from build123d import *

# Parameters (mm, degrees)
BOSS_EXTRUDE1_DEPTH    = 4.75
CUT_EXTRUDE1_REACH     = 11.471
CUT_EXTRUDE2_DEPTH     = 0.85
SKETCH6_W              = 0.8
SKETCH6_H              = 2
CUT_EXTRUDE3_DEPTH     = 0.85
SKETCH7_W              = 1.05
SKETCH7_H              = 0.85
BOSS_EXTRUDE2_DEPTH    = 1
SKETCHED_START         = 1.85
SKETCHED_BEND1_DEPTH   = 1.05
SKETCHED_BEND1_2_DEPTH = 1.05
BOSS_EXTRUDE3_DEPTH    = 0.85


# Read off the part's stored shape, not the designer's step: Sketched Bend1
with BuildPart() as part:
    # Sketch1 → Boss-Extrude1 (new body)
    with BuildSketch(Plane(origin=(0, 0, 0), x_dir=(0, 0, -1), z_dir=(1, 0, 0))):
        Polygon((0, 0.15), (0, 7.05), (-0.241393443, 8.15), (-0.647131148, 8.15), (-0.85, 7.05), (-0.85, 0.15), align=None)
    extrude(amount=BOSS_EXTRUDE1_DEPTH)

    # Cut-Extrude1: up to this face of the body (flat: up to its plane)
    cut_extrude1_end = Plane(part.part.faces().sort_by_distance((2.375, 3.6, 0))[0])
    # Sketch4 → Cut-Extrude1 (cut, up to the picked face)
    with BuildSketch(Plane.XY.offset(0.85), mode=Mode.PRIVATE) as cut_extrude1_sk1:
        Polygon((0, 6.9), (1.25, 8.15), (0, 8.15), align=None)
    cut_extrude1_tool1 = split(extrude(cut_extrude1_sk1.sketch, amount=-CUT_EXTRUDE1_REACH, mode=Mode.PRIVATE), bisect_by=cut_extrude1_end, keep=Keep.BOTH, mode=Mode.PRIVATE)
    # Sketch4 → Cut-Extrude1 (cut, up to the picked face)
    with BuildSketch(Plane.XY.offset(0.85), mode=Mode.PRIVATE) as cut_extrude1_sk2:
        Polygon((3.5, 8.15), (4.75, 6.9), (4.75, 8.15), align=None)
    cut_extrude1_tool2 = split(extrude(cut_extrude1_sk2.sketch, amount=-CUT_EXTRUDE1_REACH, mode=Mode.PRIVATE), bisect_by=cut_extrude1_end, keep=Keep.BOTH, mode=Mode.PRIVATE)
    add(cut_extrude1_tool1.solids().sort_by(Axis((0.416667, 7.733333, 0.85), (0, 0, -1)))[0], mode=Mode.SUBTRACT)
    add(cut_extrude1_tool2.solids().sort_by(Axis((4.333333, 7.733333, 0.85), (0, 0, -1)))[0], mode=Mode.SUBTRACT)

    # Sketch5 → Cut-Extrude2 (cut)
    with BuildSketch(Plane.XY.offset(0.85)):
        with BuildLine():
            Line((1.913461538, 5.842307692), (1.451923077, 4.734615385))
            ThreePointArc((1.451923077, 4.734615385), (2.37510742, 3.350000006), (3.297994271, 4.734813689))
            Line((3.297994271, 4.734813689), (2.842436975, 5.827489929))
            ThreePointArc((2.842436975, 5.827489929), (2.382974312, 6.149936406), (1.913461538, 5.842307692))
        make_face()
    extrude(amount=-CUT_EXTRUDE2_DEPTH, mode=Mode.SUBTRACT)

    # Sketch6 → Cut-Extrude3 (cut)
    with BuildSketch(Plane(origin=(0, 0, 0), x_dir=(-1, 0, 0), z_dir=(0, 0, -1))):
        with Locations((-3.3, 1.15)):
            Rectangle(SKETCH6_W, SKETCH6_H)
        with Locations((-1.45, 1.15)):
            Rectangle(SKETCH6_W, SKETCH6_H)
    extrude(amount=-CUT_EXTRUDE3_DEPTH, mode=Mode.SUBTRACT)

    # Sketch7 → Boss-Extrude2 (add)
    with BuildSketch(Plane.XZ.offset(-0.15)):
        with Locations((2.375, 0.425)):
            Rectangle(SKETCH7_W, SKETCH7_H)
    extrude(amount=BOSS_EXTRUDE2_DEPTH)

    # Sketched Bend1 outline → Sketched Bend1 (cut)
    with BuildSketch(Plane.YZ.offset(SKETCHED_START)):
        with BuildLine():
            Line((1.266116524, 0.366116524), (0.782233048, 0.85))
            Line((0.782233048, 0.85), (-0.85, 0.85))
            Line((-0.85, 0.85), (-0.85, 0))
            Line((-0.85, 0), (2.15, 0))
            ThreePointArc((2.15, 0), (1.67164571, 0.095150584), (1.266116524, 0.366116524))
        make_face()
    extrude(amount=SKETCHED_BEND1_DEPTH, mode=Mode.SUBTRACT)

    # Sketched Bend1 2 outline → Sketched Bend1 2 (add)
    with BuildSketch(Plane.YZ.offset(SKETCHED_START)):
        with BuildLine():
            ThreePointArc((2.15, 0.85), (1.996926627, 0.880448187), (1.867157288, 0.967157288))
            Line((1.867157288, 0.967157288), (0.204009247, 2.630305328))
            Line((0.204009247, 2.630305328), (-0.397031517, 2.029264564))
            Line((-0.397031517, 2.029264564), (0.782233048, 0.85))
            Line((0.782233048, 0.85), (2.15, 0.85))
        make_face()
    extrude(amount=SKETCHED_BEND1_2_DEPTH)

    # Sketch15 → Boss-Extrude3 (add)
    with BuildSketch(Plane.XY.offset(0.85)):
        Polygon((0, 2.15), (-0.50789834, 1.808617859), (-0.890356386, 0.15), (0, 0.15), align=None)
    extrude(amount=-BOSS_EXTRUDE3_DEPTH)


solid = part.part
Geometry check sheet. Reference: the model listing, model coordinates, mm. A direction names the side the tool comes from. Coordinates: 2 decimals unless noted, no trailing zeros. Order: outer loops, then holes, each group sorted by start corner. A loop starts at its lowest first (then second) coordinate and runs counter-clockwise, first axis right, second up. Notation, with made-up numbers: (4.25, 17.5) -> (58.25, 17.5) arc R20 ccw to (58.25, 50.5) -> close; hole circle Ø2 at (23, 48). An arc over 180 degrees is marked (long way). Use a Markdown table: item, result. Add a question column.
1. Cross-section at C-C (x = 2.65). Enter the section's corners in (y, z).
2. Cross-section at A-A (y = 4.35). Enter the section's corners in (x, z) (3 decimals).
3. Cross-section at B-B (z = 0.75). Enter the section's corners in (x, y) (3 decimals), and give its area (3 significant figures).
4. Set-up check for faces 1 (the face through (2.37, 1.68, 0.09)), 2 (the face through (0, 4.6, 0.4)), 3 (the face through (2.39, 6.15, 0.43)), 4 (the face through (1.05, 1.1, 0.4)): record each of +Z, -Z, +X, -X, +Y, -Y from which the full face is reachable in a straight line by a thin tool's end or side.
5. Go/stop test with flat-tipped pins: pin 1 Ø0.9 at (x, z) = (3.5, 0.5) entering from -Y; pin 2 Ø1.5 at (x, y) = (2.5, 5.5) entering from +Z. Record where each tip stops, or that it passes through.
6. Cross-section at D-D (y = 6.25). Enter the section's corners in (x, z), and give its area (3 significant figures).
7. Mould release check, pull along X, two halves, no side actions. Record for faces 5 (the face through (4.26, 7.39, 0.43)), 6 (the face through (1, 4, 0)), 7 (the face through (1.5, 2.15, 0.4)), 8 (the face through (2.9, 1, 1)): pulls with the +X half, pulls with the -X half, needs draft (parallel to the pull), parting line crosses it, or undercut.
8. Material ranges on L1, parallel to X at y = 4.35, z = 0.5 (3 decimals); L2, parallel to Z at x = 4.4, y = 5; L3, parallel to Y at x = 0.95, z = 0.55, recorded low to high.
Filled sheet:
| question | item | result |
|---|---|---|
| 1 | outline | (-0.4, 2.03) -> (1.27, 0.37) arc R1.25 ccw to (2.15, 0) -> (3.39, 0) -> (3.39, 0.85) -> (2.15, 0.85) arc R0.4 cw to (1.87, 0.97) -> (0.2, 2.63) -> close; (6.07, 0) -> (7.05, 0) -> (8.15, 0.24) -> (8.15, 0.65) -> (7.05, 0.85) -> (6.07, 0.85) -> close |
| 2 | outline | (0, 0) -> (1.375, 0) -> (1.375, 0.85) -> (0, 0.85) -> close; (3.375, 0) -> (4.75, 0) -> (4.75, 0.85) -> (3.375, 0.85) -> close |
| 3 | outline | (-0.89, 0.15) -> (1.05, 0.15) -> (1.05, 2.15) -> (1.85, 2.15) -> (1.85, 0.882) -> (2.9, 0.882) -> (2.9, 2.15) -> (3.7, 2.15) -> (3.7, 0.15) -> (4.75, 0.15) -> (4.75, 6.9) -> (4.058, 7.592) -> (0.692, 7.592) -> (0, 6.9) -> (0, 2.15) -> (-0.508, 1.809) -> close; hole (1.452, 4.735) arc R1 ccw (long way) to (3.298, 4.735) -> (2.842, 5.827) arc R0.5 ccw to (1.913, 5.842) -> close |
| 3 | area | 28.1 mm2 |
| 4 | face 1 | -Z, -Y |
| 4 | face 2 | +Z, -Z, -X, +Y |
| 4 | face 3 | +Z, -Z |
| 4 | face 4 | +Z, -Z, -Y |
| 5 | pin 1 | y = 0.15 |
| 5 | pin 2 | z = 0.85 |
| 6 | outline | (0, 0) -> (4.75, 0) -> (4.75, 0.85) -> (0, 0.85) -> close |
| 6 | area | 4.04 mm2 |
| 7 | face 5 | pulls with the +X half |
| 7 | face 6 | needs draft |
| 7 | face 7 | undercut |
| 7 | face 8 | undercut |
| 8 | L1 | 0 to 1.375, 3.375 to 4.75 |
| 8 | L2 | 0 to 0.85 |
| 8 | L3 | 0.15 to 7.85 |
